Can you work these out from the drawing? Everything is in mm from the part's minimum corner. A direction names the side the tool comes from. Round coordinates to 2 decimals unless told otherwise and drop trailing zeros. Order: outer loops, then holes, each group sorted by start corner. A loop starts at its lowest first (then second) coordinate and runs counter-clockwise, first axis right, second up. Notation, with made-up numbers: (89, 38.25) - (123, 38.25) arc R24 ccw to (123, 65.25) - close; hole circle Ø11 at (33.5, 0.5). An arc over 180 degrees is marked (long way). Answer as a JSON object with one key per item and string values.
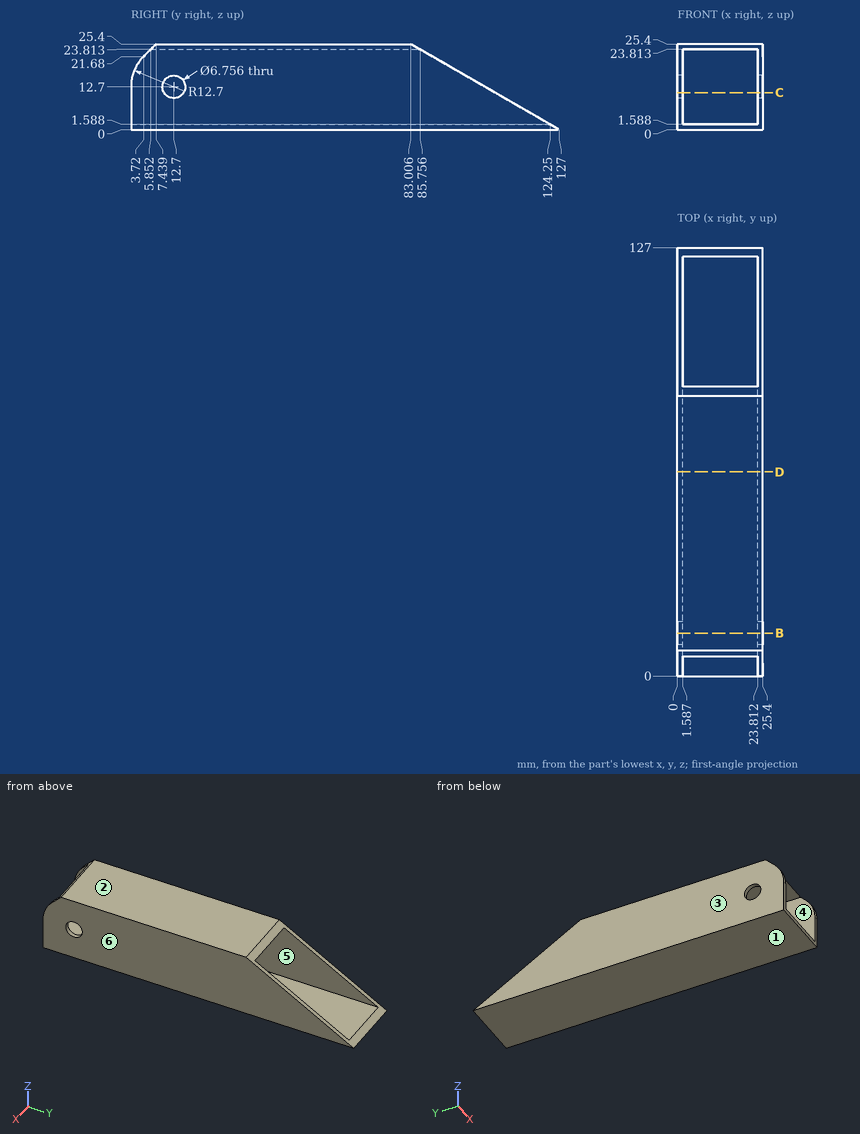
1. Imagine slicing it at B-B (y = 12.7). List the corners of the cut face in (x, z) for me, plus the area to 3 significant figures.
Responses:
{"outline": "(0, 0) - (25.4, 0) - (25.4, 9.32) - (23.81, 9.32) - (23.81, 1.59) - (1.59, 1.59) - (1.59, 9.32) - (0, 9.32) - close; (0, 16.08) - (1.59, 16.08) - (1.59, 23.81) - (23.81, 23.81) - (23.81, 16.08) - (25.4, 16.08) - (25.4, 25.4) - (0, 25.4) - close", "area": "130 mm2"}
2. If I drill on L1, parallel to X at y = 25.5, z = 2; L2, parallel to Z at x = 14, y = 100, over which ranges is the centre line in solid material (lowest first)? Write a range as [from, to].
Responses:
{"L1": "[0, 1.59], [23.81, 25.4]", "L2": "[0, 1.59]"}
3. Thinking about a two-plate mould opening in Z: for the marked faces 1, 2, 3 and 4, which applies, pulls with the +Z half, pulls with the -Z half, needs draft (parallel to the pull), parting line crosses it, or undercut?
Responses:
{"face 1": "pulls with the -Z half", "face 2": "pulls with the +Z half", "face 3": "needs draft", "face 4": "undercut"}
4. Imagine slicing it at C-C (z = 11). List the corners of the cut face in (x, y) for me.
Responses:
{"outline": "(0, 0) - (1.59, 0) - (1.59, 9.78) - (0, 9.78) - close; (0, 15.62) - (1.59, 15.62) - (1.59, 107.95) - (0, 107.95) - close; (23.81, 0) - (25.4, 0) - (25.4, 9.78) - (23.81, 9.78) - close; (23.81, 15.62) - (25.4, 15.62) - (25.4, 107.95) - (23.81, 107.95) - close"}
5. Imagine slicing it at D-D (y = 60.5). List the corners of the cut face in (x, z) for me.
Responses:
{"outline": "(0, 0) - (25.4, 0) - (25.4, 25.4) - (0, 25.4) - close; hole (1.59, 1.59) - (23.81, 1.59) - (23.81, 23.81) - (1.59, 23.81) - close"}
6. For the marked faces 5 and 6, which set-ups out of +Z, -Z, +X, -X, +Y, -Y let a thin tool reach every point of the face, with its end or its side?
Responses:
{"face 5": "+Y, -Y", "face 6": "+Z, -Z, +X, +Y, -Y"}
7. For P1, Ø10, axis at x = 21.5, z = 21, coming from the -Y side, with a flat end and sliding along its axis, tell me the tip position at first contact or that it passes through.
Responses:
{"P1": "y = 0.6"}
